from build123d import *

# Parameters (mm, degrees)
SKETCH1_R           = 2.25
BOSS_EXTRUDE1_DEPTH = 8
SKETCH2_R           = 4.525
CUT_EXTRUDE1_DEPTH  = 4
CUT_EXTRUDE2_DEPTH  = 2.5


with BuildPart() as part:
    # Sketch1 → Boss-Extrude1 (new body)
    with BuildSketch(Plane.XY):
        with BuildLine():
            Line((10, 0), (10, 108))
            ThreePointArc((10, 108), (0, 118), (-10, 108))
            Line((-10, 108), (-10, 0))
            ThreePointArc((-10, 0), (0, -10), (10, 0))
        make_face()
        Circle(SKETCH1_R, mode=Mode.SUBTRACT)
        with Locations((0, 108)):
            Circle(SKETCH1_R, mode=Mode.SUBTRACT)
    extrude(amount=BOSS_EXTRUDE1_DEPTH)

    # Sketch2 → Cut-Extrude1 (cut)
    with BuildSketch(Plane.XY.offset(8)):
        Circle(SKETCH2_R)
        with Locations((0, 108)):
            Circle(SKETCH2_R)
    extrude(amount=-CUT_EXTRUDE1_DEPTH, mode=Mode.SUBTRACT)

    # Sketch3 → Cut-Extrude2 (cut)
    with BuildSketch(Plane.XY):
        with BuildLine():
            Line((7.5, 12), (7.5, 96))
            ThreePointArc((7.5, 96), (0, 93.849028302), (-7.5, 96))
            Line((-7.5, 96), (-7.5, 12))
            ThreePointArc((-7.5, 12), (0, -14.150971698), (7.5, 12))
        make_face()
    extrude(amount=CUT_EXTRUDE2_DEPTH, mode=Mode.SUBTRACT)


solid = part.part
Could you check a few things on this model? Use its own coordinates, in mm. A direction names the side the tool comes from. Give positions to 0.01 mm unless a question says otherwise; leave off trailing zeros. Order: outer loops, then holes, each group sorted by start corner. A loop starts at its lowest first (then second) coordinate and runs counter-clockwise, first axis right, second up.
1. Will these pins go through, and if not, where does the flat tip stop? P1, Ø5, axis at x = 0, y = 0, coming from the +Z side; P2, Ø10, axis at x = -1, y = 107, coming from the +Z side; P3, Ø1.5, axis at x = -1, y = 17.5, coming from the -Z side; P4, Ø1, axis at x = 3.5, z = 1, coming from the -Y side.
2. Suppose I cut it at D-D (x = -6). List the corners of the cut face in (y, z) for me.
3. We'd pull the mould along X, two halves only. Please class faces 4 (the flat face through (-10, 55, 4)), 5 (the cylindrical face through (0, -10, 5)), 6 (the cylindrical face through (0.11, 93.85, 1.23)): pulls with the +X half, pulls with the -X half, needs draft (parallel to the pull), parting line crosses it, or undercut.
4. Suppose I cut it at B-B (y = 65.5). List the corners of the cut face in (x, z) for me.
5. For faces 1 (the flat face through (7.5, 53, 1)), 2 (the cylindrical face through (-0.29, 2.23, 3.24)), 3 (the cylindrical face through (-0.589, 112.486, 6.028)), which set-ups out of +Z, -Z, +X, -X, +Y, -Y let a thin tool reach every point of the face, with its end or its side?
6. Suppose I cut it at A-A (x = 0). List the corners of the cut face in (y, z) for me (3 decimals).
7. Suppose I cut it at C-C (z = 5.5). List the corners of the cut face in (x, y) for me (3 decimals), plus the area to 3 significant figures.
8. I need wall thicknesses on L1, parallel to Y at x = 0, z = 4.9 (3 decimals); L2, parallel to X at y = 45, z = 1.25; L3, parallel to X at y = 108, z = 3.1. Which ranges of each line are inside material? Lowest first, please.
Solved:
1. P1: stops at z = 4
1. P2: stops at z = 8
1. P3: stops at z = 2.5
1. P4: stops at y = 94.17
2. outline: (-8, 2.5) - (95.18, 2.5) - (95.18, 0) - (116, 0) - (116, 8) - (-8, 8) - close
3. face 4: pulls with the -X half
3. face 5: parting line crosses it
3. face 6: undercut
4. outline: (-10, 0) - (-7.5, 0) - (-7.5, 2.5) - (7.5, 2.5) - (7.5, 0) - (10, 0) - (10, 8) - (-10, 8) - close
5. face 1: -Z, -Y
5. face 2: +Z, -Z
5. face 3: +Z
6. outline: (-10, 2.5) - (-2.25, 2.5) - (-2.25, 4) - (-4.525, 4) - (-4.525, 8) - (-10, 8) - close; (2.25, 2.5) - (93.849, 2.5) - (93.849, 0) - (105.75, 0) - (105.75, 4) - (103.475, 4) - (103.475, 8) - (4.525, 8) - (4.525, 4) - (2.25, 4) - close; (110.25, 0) - (118, 0) - (118, 8) - (112.525, 8) - (112.525, 4) - (110.25, 4) - close
7. outline: (-10, 0) arc R10 ccw to (10, 0) - (10, 108) arc R10 ccw to (-10, 108) - close; hole circle Ø9.05 at (0, 0); hole circle Ø9.05 at (0, 108)
7. area: 2,350 mm2
8. L1: y = -10 to -4.525, 4.525 to 103.475, 112.525 to 118
8. L2: x = -10 to -7.5, 7.5 to 10
8. L3: x = -10 to -2.25, 2.25 to 10
